Build history of the part. All positions in model axes, mm. Give positions to 0.01 mm unless a question says otherwise; leave off trailing zeros. Order: outer loops, then holes, each group sorted by start corner. A loop starts at its lowest first (then second) coordinate and runs counter-clockwise, first axis right, second up. Notation, with made-up numbers: (-8.5, 12.25) - (20.5, 12.25) arc R25 cw to (20.5, 44.25) - close; hole circle Ø11 at (-1, 66.5). An arc over 180 degrees is marked (long way). One line per item, written item: value.
```python
from build123d import *

# Parameters (mm, degrees)
CROQUIS1_W              = 40
CROQUIS1_H              = 17
SALIENTE_EXTRUIR1_DEPTH = 5
CORTAR_EXTRUIR1_DEPTH   = 40
SALIENTE_EXTRUIR2_DEPTH = 17
CORTAR_EXTRUIR2_DEPTH   = 17
SALIENTE_EXTRUIR3_DEPTH = 17


with BuildPart() as part:
    # Croquis1 → Saliente-Extruir1 (new body)
    with BuildSketch(Plane(origin=(0, 0, 0), x_dir=(1, 0, 0), z_dir=(0, 1, 0))):
        Rectangle(CROQUIS1_W, CROQUIS1_H)
    extrude(amount=SALIENTE_EXTRUIR1_DEPTH)

    # Croquis2 → Cortar-Extruir1 (cut)
    with BuildSketch(Plane.XY.offset(8.5)):
        Polygon((-20, 5), (-20, 0), (-10, 0), (-5, 5), align=None)
    extrude(amount=-CORTAR_EXTRUIR1_DEPTH, mode=Mode.SUBTRACT)

    # Croquis3 → Saliente-Extruir2 (add)
    with BuildSketch(Plane(origin=(0, 0, -8.5), x_dir=(-1, 0, 0), z_dir=(0, 0, -1))):
        Polygon((10, 5), (10, 0), (5, 5), align=None)
    extrude(amount=-SALIENTE_EXTRUIR2_DEPTH)

    # Croquis4 → Cortar-Extruir2 (cut)
    with BuildSketch(Plane(origin=(0, 0, -8.5), x_dir=(-1, 0, 0), z_dir=(0, 0, -1))):
        Polygon((10, 5), (0, 0), (10, 0), align=None)
    extrude(amount=-CORTAR_EXTRUIR2_DEPTH, mode=Mode.SUBTRACT)

    # Croquis5 → Saliente-Extruir3 (add)
    with BuildSketch(Plane(origin=(0, 0, -8.5), x_dir=(-1, 0, 0), z_dir=(0, 0, -1))):
        Polygon((-20, 5), (-30, 5), (-20, 0), align=None)
    extrude(amount=-SALIENTE_EXTRUIR3_DEPTH)


solid = part.part
```
(1) Slice it at A-A, the plane y = 1.3. Give the cut face in (x, z).
Completed:
outline: (-2.6, -8.5) - (22.6, -8.5) - (22.6, 8.5) - (-2.6, 8.5) - close
(2) Slice it at B-B, the plane x = 21. Give the cut face in (y, z).
Completed:
outline: (0.5, -8.5) - (5, -8.5) - (5, 8.5) - (0.5, 8.5) - close
(3) Drill centre lines: line 1 (X direction, y = 4.55, z = -4); line 2 (Y direction, x = 23, z = -7); line 3 (Y direction, x = -7, z = 0.75). Where is each one in solid material? Low to high.
Completed:
line 1: -9.1 to 29.1
line 2: 1.5 to 5
line 3: 3.5 to 5
(4) Pin check, flat tips, straight feed: P1, Ø1.5, axis at x = 10.5, z = 5, coming from the -Y side; P2, Ø3, axis at y = 3, z = -2, coming from the -X side. Stop position of each tip, or through.
Completed:
P1: y = 0
P2: x = -9
